Here's how the part is built. I have some questions about the finished solid (model axes, mm). A direction names the side the tool comes from. Give positions to 0.01 mm unless a question says otherwise; leave off trailing zeros. Loops run counter-clockwise (first coordinate to the right, second up) from the corner with the lowest first, then second, coordinate; pieces in that order, holes last. Notation, with made-up numbers: (25.25, -21) - (48.25, -21) arc R16 ccw to (48.25, 8) - close; hole circle Ø1 at (18.25, 15). An arc over 180 degrees is marked (long way). Use a Markdown table: item, result.
from build123d import *

# Parameters (mm, degrees)
SKETCH1_W           = 50.8
SKETCH1_H           = 25.4
BOSS_EXTRUDE1_DEPTH = 19.05
SKETCH4_W           = 10.16
SKETCH4_H           = 3.054556314
CUT_EXTRUDE2_DEPTH  = 19.05
SKETCH5_W           = 10.16
SKETCH5_H           = 3.175
CUT_EXTRUDE3_DEPTH  = 17.78
SKETCH6_R           = 1.5
CUT_EXTRUDE4_DEPTH  = 10.16
CUT_EXTRUDE5_START  = -10.16
SKETCH7_R           = 1.5
CUT_EXTRUDE5_DEPTH  = 10.16
SKETCH8_R           = 1.5
CUT_EXTRUDE6_DEPTH  = 10.16


with BuildPart() as part:
    # Sketch1 → Boss-Extrude1 (new body)
    with BuildSketch(Plane.XY):
        Rectangle(SKETCH1_W, SKETCH1_H)
    extrude(amount=BOSS_EXTRUDE1_DEPTH)

    # Sketch4 → Cut-Extrude2 (cut)
    with BuildSketch(Plane(origin=(0, 12.7, 0), x_dir=(1, 0, 0), z_dir=(0, 1, 0))):
        with Locations((0, -16.252721843)):
            Rectangle(SKETCH4_W, SKETCH4_H)
    extrude(amount=-CUT_EXTRUDE2_DEPTH, mode=Mode.SUBTRACT)

    # Sketch5 → Cut-Extrude3 (cut)
    with BuildSketch(Plane(origin=(0, 0, 0), x_dir=(-1, 0, 0), z_dir=(0, 0, -1))):
        with Locations((0, -7.9375)):
            Rectangle(SKETCH5_W, SKETCH5_H)
    extrude(amount=-CUT_EXTRUDE3_DEPTH, mode=Mode.SUBTRACT)

    # Sketch6 → Cut-Extrude4 (cut)
    with BuildSketch(Plane.ZY.offset(25.4)):
        with Locations((9.525, -7.62)):
            Circle(SKETCH6_R)
        with Locations((9.525, 7.62)):
            Circle(SKETCH6_R)
    extrude(amount=-CUT_EXTRUDE4_DEPTH, mode=Mode.SUBTRACT)

    # Sketch7 → Cut-Extrude5 (cut)
    with BuildSketch(Plane(origin=(25.4, 0, 0), x_dir=(0, 0, -1), z_dir=(1, 0, 0)).offset(CUT_EXTRUDE5_START)):
        with Locations(Location((-9.525, 7.62, 0), (0, 0, 180))):
            Circle(SKETCH7_R)
        with Locations(Location((-9.525, -7.62, 0), (0, 0, 180))):
            Circle(SKETCH7_R)
    extrude(amount=CUT_EXTRUDE5_DEPTH, mode=Mode.SUBTRACT)

    # Sketch8 → Cut-Extrude6 (cut)
    with BuildSketch(Plane(origin=(0, 0, 0), x_dir=(-1, 0, 0), z_dir=(0, 0, -1))):
        with Locations((22.225, 0)):
            Circle(SKETCH8_R)
        with Locations((-22.225, 0)):
            Circle(SKETCH8_R)
    extrude(amount=-CUT_EXTRUDE6_DEPTH, mode=Mode.SUBTRACT)


solid = part.part
(1) Suppose I cut it at B-B on z = 6.25. Write out the boundary of the cut face in (x, y) (3 decimals).
A:
| item | result |
|---|---|
| outline | (-25.4, -12.7) - (25.4, -12.7) - (25.4, 12.7) - (-25.4, 12.7) - close; hole circle Ø3 at (-22.225, 0); hole (-5.08, -9.525) - (5.08, -9.525) - (5.08, -6.35) - (-5.08, -6.35) - close; hole circle Ø3 at (22.225, 0) |
(2) Suppose I cut it at C-C on x = -16. Write out the boundary of the cut face in (y, z) (3 decimals), plus the area to 3 significant figures.
A:
| item | result |
|---|---|
| outline | (-12.7, 0) - (12.7, 0) - (12.7, 19.05) - (-12.7, 19.05) - close; hole circle Ø3 at (-7.62, 9.525); hole circle Ø3 at (7.62, 9.525) |
| area | 470 mm2 |
(3) Will these pins go through, and if not, where does the flat tip stop? pin 1 (0.9 mm diameter, centred on y = -7, z = 9, fed in from -X); pin 2 (1.5 mm diameter, centred on y = 7.5, z = 10, fed in from +X); pin 3 (2.5 mm diameter, centred on x = 22.225, y = 0, fed in from -Z).
A:
| item | result |
|---|---|
| pin 1 | x = -15.24 |
| pin 2 | x = 15.24 |
| pin 3 | z = 10.16 |
(4) Suppose I cut it at A-A on y = 0. Write out the boundary of the cut face in (x, z) (3 decimals), plus the area to 3 significant figures.
A:
| item | result |
|---|---|
| outline | (-25.4, 0) - (-23.725, 0) - (-23.725, 10.16) - (-20.725, 10.16) - (-20.725, 0) - (20.725, 0) - (20.725, 10.16) - (23.725, 10.16) - (23.725, 0) - (25.4, 0) - (25.4, 19.05) - (-25.4, 19.05) - close; hole (-5.08, 14.725) - (5.08, 14.725) - (5.08, 17.78) - (-5.08, 17.78) - close |
| area | 876 mm2 |
(5) On a 3-axis mill with a long thin cutter (end or side, diameter ignored), from which of +Z, -Z, +X, -X, +Y, -Y can I reach the whole of each face in a straight line? I mean faces 1 (the face through (0, -9.525, 9)), 2 (the face through (0, 2, 17.78)), 3 (the face through (5.08, -2, 15)), 4 (the face through (20.249, -6.707, 8.335)), 5 (the face through (-15.24, 8, 10)). Say none if no direction works.
A:
| item | result |
|---|---|
| face 1 | -Z |
| face 2 | +Y |
| face 3 | none |
| face 4 | +X |
| face 5 | -X |
(6) Suppose I cut it at D-D on y = -7.62. Write out the boundary of the cut face in (x, z) (3 decimals), plus the area to 3 significant figures.
A:
| item | result |
|---|---|
| outline | (-25.4, 0) - (-5.08, 0) - (-5.08, 17.78) - (5.08, 17.78) - (5.08, 0) - (25.4, 0) - (25.4, 8.025) - (15.24, 8.025) - (15.24, 11.025) - (25.4, 11.025) - (25.4, 19.05) - (-25.4, 19.05) - (-25.4, 11.025) - (-15.24, 11.025) - (-15.24, 8.025) - (-25.4, 8.025) - close |
| area | 726 mm2 |
(7) We'd pull the mould along Z, two halves only. Please class faces 6 (the face through (0, -12.7, 9)), 7 (the face through (0, 0, 0)), 8 (the face through (15.24, -8, 10)): pulls with the +Z half, pulls with the -Z half, needs draft (parallel to the pull), parting line crosses it, or undercut.
A:
| item | result |
|---|---|
| face 6 | needs draft |
| face 7 | pulls with the -Z half |
| face 8 | undercut |
(8) If I drill on line 1 (X direction, y = 0.5, z = 9.25); line 2 (Y direction, x = -5, z = 2.75) (3 decimals); line 3 (X direction, y = 0.75, z = 6.75), over which ranges is the centre line in solid material (lowest first)?
A:
| item | result |
|---|---|
| line 1 | -25.4 to -23.64, -20.81 to 20.81, 23.64 to 25.4 |
| line 2 | -12.7 to -9.525, -6.35 to 12.7 |
| line 3 | -25.4 to -23.52, -20.93 to 20.93, 23.52 to 25.4 |
